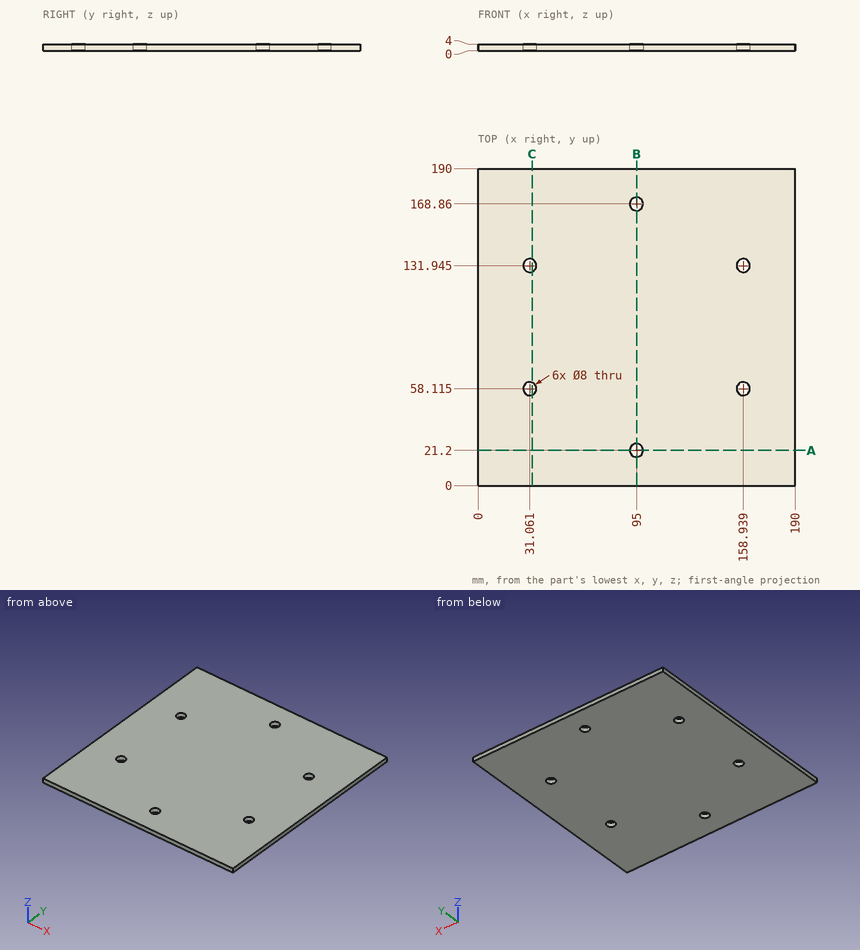
Could you check a few things on this drawing? It's one solid part, dimensions in mm from its lowest x, y, z. Coordinates: 2 decimals unless noted, no trailing zeros. Write each loop counter-clockwise with the first axis right and the second up, starting at its lowest first coordinate (ties: lowest second). Pieces come first, ordered by that corner, then holes. Notation, with made-up numbers: (46.25, 67.5) - (97.25, 67.5) arc R12 ccw to (97.25, 76.5) - close; hole circle Ø10 at (33.5, 20). An arc over 180 degrees is marked (long way). Use one line per item in the form item = value.
1) Suppose I cut it at A-A, the plane y = 21.2. Write out the boundary of the cut face in (x, z), plus the area to 3 significant figures.
Solved:
outline = (0, 0) - (91, 0) - (91, 4) - (0, 4) - close; (99, 0) - (190, 0) - (190, 4) - (99, 4) - close
area = 728 mm2
2) Suppose I cut it at C-C, the plane x = 32.5. Write out the boundary of the cut face in (y, z).
Solved:
outline = (0, 0) - (54.38, 0) - (54.38, 4) - (0, 4) - close; (61.85, 0) - (128.21, 0) - (128.21, 4) - (61.85, 4) - close; (135.68, 0) - (190, 0) - (190, 4) - (135.68, 4) - close
3) I need wall thicknesses on line 1 (Y direction, x = 95, z = 1.35); line 2 (Y direction, x = 98.5, z = 3.5) (1 decimal); line 3 (X direction, y = 133.5, z = 1.3) (1 decimal). Which ranges of each line are inside material? Lowest first, please.
Solved:
line_1 = 0 to 17.2, 25.2 to 164.86, 172.86 to 190
line_2 = 0 to 19.3, 23.1 to 166.9, 170.8 to 190
line_3 = 0 to 27.4, 34.7 to 155.3, 162.6 to 190
4) I'm going to push a flat-ended pin straight in: P1, Ø5, axis at x = 158.94, y = 58.12, coming from the -Z side. Where does the tip first touch, or does it pass through?
Solved:
P1 = through
5) Suppose I cut it at B-B, the plane x = 95. Write out the boundary of the cut face in (y, z).
Solved:
outline = (0, 0) - (17.2, 0) - (17.2, 4) - (0, 4) - close; (25.2, 0) - (164.86, 0) - (164.86, 4) - (25.2, 4) - close; (172.86, 0) - (190, 0) - (190, 4) - (172.86, 4) - close
